Work out the finished part from the listing and answer in its coordinate system (mm). Face numbers are marked on the shaded views. A direction names the side the tool comes from. Coordinates: 2 decimals unless noted, no trailing zeros. Order: outer loops, then holes, each group sorted by start corner. A loop starts at its lowest first (then second) coordinate and runs counter-clockwise, first axis right, second up. Notation, with made-up numbers: (11, 71) - (60, 71) arc R24 ccw to (60, 101) - close; hole circle Ø7 at (18.5, 45.5). An arc over 180 degrees is marked (long way). Answer as a JSON object with one key per item and string values. Group by question number.
1) Section D-D (y = 120.5) is taken. Give the vertices of the cut face in (x, z), plus the area to 3 significant figures.
2) The mould has two halves that part along Z. Classify the marked faces 1, 2 and 3: released by +Z, released by -Z, zero draft, split by the parting line, or undercut.
3) Section A-A (x = 25.4) is taken. Give the vertices of the cut face in (y, z).
4) Find the intervals of material crossed by line 1 along X through (y, z) = (13, 6); line 2 along X through (y, z) = (112, 25.4); line 3 along X through (y, z) = (45, 25), in increasing order.
5) Section C-C (y = 61) is taken. Give the vertices of the cut face in (x, z).
6) A tool of negligible diameter and unlimited length cuts with its end or side. For the marked faces 4 and 5, from which of +Z, -Z, +X, -X, +Y, -Y can it reach the whole face along a straight path? Write none if from no direction.
7) Section B-B (z = 25.4) is taken. Give the vertices of the cut face in (x, y) (3 decimals), plus the area to 3 significant figures.
8) Each of these flat-tipped pins is pushed along its axis until it touches: P1, Ø14.5, axis at x = 26.5, z = 25, coming from the -Y side; P2, Ø14, axis at x = 25.4, z = 25.4, coming from the +Y side; P3, Ø1.5, axis at x = 16.5, z = 28.5, coming from the -Y side. Where does it stop, or does it pass through?
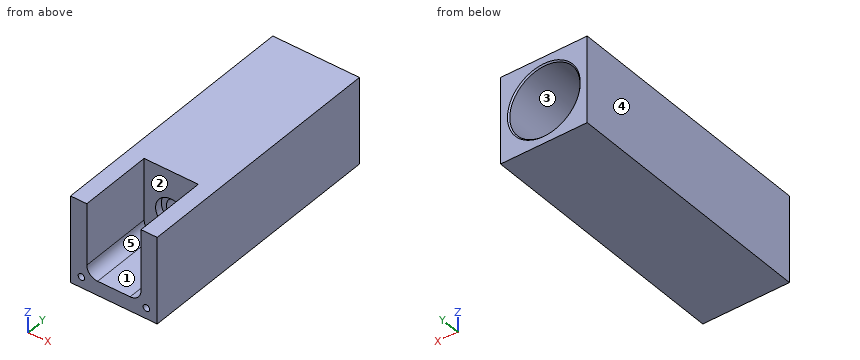
from build123d import *

# Parameters (mm, degrees)
SKETCH1_W                  = 50.8
SKETCH1_H                  = 50.8
BOSS_EXTRUDE1_DEPTH        = 152.4
SKETCH2_R                  = 6.1468
CUT_EXTRUDE1_DEPTH         = 153.4
SKETCH3_R                  = 20.5994
CUT_EXTRUDE2_DEPTH         = 74.93
SKETCH4_R                  = 17.78
CUT_EXTRUDE3_DEPTH         = 82.55
CUT_EXTRUDE4_DEPTH         = 42.4434
SKETCH6_R                  = 9.144
CUT_EXTRUDE5_DEPTH         = 4.318
FILLET1_R                  = 6.35
F_10_24_TAPPED_HOLE1_D     = 3.7973
F_10_24_TAPPED_HOLE1_DEPTH = 17.78
F_10_24_TAPPED_HOLE1_TIP   = 1.140824014
CHAMFER1_SIZE              = 0.762


with BuildPart() as part:
    # Sketch1 → Boss-Extrude1 (new body)
    with BuildSketch(Plane(origin=(0, 0, 0), x_dir=(1, 0, 0), z_dir=(0, 1, 0))):
        with Locations((25.4, -25.4)):
            Rectangle(SKETCH1_W, SKETCH1_H)
    extrude(amount=BOSS_EXTRUDE1_DEPTH)

    # Sketch2 → Cut-Extrude1 (cut, through all)
    with BuildSketch(Plane(origin=(0, 152.4, 0), x_dir=(1, 0, 0), z_dir=(0, 1, 0))):
        with Locations((25.4, -25.4)):
            Circle(SKETCH2_R)
    extrude(amount=-CUT_EXTRUDE1_DEPTH, mode=Mode.SUBTRACT)

    # Sketch3 → Cut-Extrude2 (cut)
    with BuildSketch(Plane(origin=(0, 152.4, 0), x_dir=(1, 0, 0), z_dir=(0, 1, 0))):
        with Locations((25.4, -25.4)):
            Circle(SKETCH3_R)
    extrude(amount=-CUT_EXTRUDE2_DEPTH, mode=Mode.SUBTRACT)

    # Sketch4 → Cut-Extrude3 (cut)
    with BuildSketch(Plane(origin=(0, 152.4, 0), x_dir=(1, 0, 0), z_dir=(0, 1, 0))):
        with Locations((25.4, -25.4)):
            Circle(SKETCH4_R)
    extrude(amount=-CUT_EXTRUDE3_DEPTH, mode=Mode.SUBTRACT)

    # Sketch5 → Cut-Extrude4 (cut)
    with BuildSketch(Plane.XY.offset(50.8)):
        Polygon((9.525, 0), (9.525, 36.83), (9.525, 43.18), (15.875, 43.18), (34.925, 43.18), (41.275, 43.18), (41.275, 36.83), (41.275, 0), align=None)
    extrude(amount=-CUT_EXTRUDE4_DEPTH, mode=Mode.SUBTRACT)

    # Sketch6 → Cut-Extrude5 (cut)
    with BuildSketch(Plane.XZ.offset(-43.18)):
        with Locations((25.4, 25.4)):
            Circle(SKETCH6_R)
    extrude(amount=-CUT_EXTRUDE5_DEPTH, mode=Mode.SUBTRACT)

    # Fillet1
    fillet1_edges = [part.edges().sort_by_distance(p)[0] for p in [
        (9.525, 21.59, 8.3566),
        (41.275, 21.59, 8.3566),
    ]]
    fillet(fillet1_edges, radius=FILLET1_R)

    # #10-24 Tapped Hole1
    with Locations(Plane(origin=(0, 0, 0), x_dir=(-1, 0, 0), z_dir=(0, -1, 0))):
        with Locations((-6.35, -6.35), (-44.45, -6.35)):
            Hole(F_10_24_TAPPED_HOLE1_D / 2, depth=F_10_24_TAPPED_HOLE1_DEPTH)
            with Locations((0, 0, -(F_10_24_TAPPED_HOLE1_DEPTH + F_10_24_TAPPED_HOLE1_TIP / 2))):  # 118° drill point
                Cone(0, F_10_24_TAPPED_HOLE1_D / 2, F_10_24_TAPPED_HOLE1_TIP, mode=Mode.SUBTRACT)

    # Chamfer1
    chamfer1_edges = [part.edges().sort_by_distance(p)[0] for p in [
        (4.8006, 152.4, 25.4),
    ]]
    chamfer(chamfer1_edges, length=CHAMFER1_SIZE)


solid = part.part
Report:
{
 "1": {"outline": "(0, 0) - (50.8, 0) - (50.8, 50.8) - (0, 50.8) - close; hole circle Ø41.2 at (25.4, 25.4)", "area": "1,250 mm²"},
 "2": {"face 1": "released by +Z", "face 2": "zero draft", "face 3": "undercut"},
 "3": {"outline": "(0, 0) - (152.4, 0) - (152.4, 4.04) - (151.64, 4.8) - (77.47, 4.8) - (77.47, 7.62) - (69.85, 7.62) - (69.85, 19.25) - (47.5, 19.25) - (47.5, 16.26) - (43.18, 16.26) - (43.18, 8.36) - (0, 8.36) - close; (43.18, 34.54) - (47.5, 34.54) - (47.5, 31.55) - (69.85, 31.55) - (69.85, 43.18) - (77.47, 43.18) - (77.47, 46) - (151.64, 46) - (152.4, 46.76) - (152.4, 50.8) - (43.18, 50.8) - close"},
 "4": {"line 1": "x = 0 to 4.48, 8.22 to 42.58, 46.32 to 50.8", "line 2": "x = 0 to 4.8, 46 to 50.8", "line 3": "x = 0 to 16.26, 34.54 to 50.8"},
 "5": {"outline": "(0, 0) - (50.8, 0) - (50.8, 50.8) - (0, 50.8) - close; hole circle Ø12.29 at (25.4, 25.4)"},
 "6": {"face 4": "+Z, -Z, -X, +Y, -Y", "face 5": "+Z, -Y"},
 "7": {"outline": "(0, 0) - (9.525, 0) - (9.525, 43.18) - (16.256, 43.18) - (16.256, 47.498) - (19.253, 47.498) - (19.253, 69.85) - (7.62, 69.85) - (7.62, 77.47) - (4.801, 77.47) - (4.801, 151.638) - (4.039, 152.4) - (0, 152.4) - close; (31.547, 47.498) - (34.544, 47.498) - (34.544, 43.18) - (41.275, 43.18) - (41.275, 0) - (50.8, 0) - (50.8, 152.4) - (46.761, 152.4) - (45.999, 151.638) - (45.999, 77.47) - (43.18, 77.47) - (43.18, 69.85) - (31.547, 69.85) - close", "area": "2,660 mm²"},
 "8": {"P1": "stops at y = 47.5", "P2": "stops at y = 69.85", "P3": "stops at y = 43.18"}
}
